The listing builds one solid part. Answer for the finished solid, in the listing's coordinates (mm). A direction names the side the tool comes from. Coordinates: 2 decimals unless noted, no trailing zeros. Loops run counter-clockwise (first coordinate to the right, second up) from the corner with the lowest first, then second, coordinate; pieces in that order, holes last. Notation, with made-up numbers: (33, 72) -> (43, 72) arc R27 ccw to (43, 95) -> close; hole circle Ø2 at (29.25, 46). An arc over 180 degrees is marked (long way). Answer in a Markdown table with one row per item.
```python
from build123d import *

# Parameters (mm, degrees)
F1_DEPTH = 41.95
F3_DEPTH = 39.95
F5_DEPTH = 5


with BuildPart() as f1:
    # F0 (on Front) → F1 (new body)
    with BuildSketch(Plane.XZ):
        Polygon((54.9357536622, -12.7440134094), (54.9357536622, 0.0059865906), (54.9357536622, 12.7559865906), (-52.01294007, 22.7216603247), (-52.0118536268, -22.7213396623), align=None)
    extrude(amount=F1_DEPTH)

    # F2 (on face) → F3 (cut)
    with BuildSketch(Plane.XZ.offset(41.95)):
        Polygon((54.9357536622, 10.7559865906), (-52.0128922544, 20.7216603253), (-52.0119014425, -20.7213396629), (54.9357536622, -10.7440134094), align=None)
    extrude(amount=-F3_DEPTH, mode=Mode.SUBTRACT)

    # F4 (on face) → F5 (cut)
    with BuildSketch(Plane.XZ.offset(2)):
        Polygon((-17.6542899587, 4.4775479473), (-22.824516984, 4.4775479473), (-25.4096304967, 0), (-22.824516984, -4.4775479473), (-17.6542899587, -4.4775479473), (-15.069176446, 0), align=None)
        Polygon((4.0099493481, -2.841678097), (4.4659400954, 2.0518789548), (0.4559907474, 4.8935570518), (-4.0099493481, 2.841678097), (-4.4659400954, -2.0518789548), (-0.4559907474, -4.8935570518), align=None)
        Polygon((24.5754495263, 0.2760817257), (21.8509733677, 4.442849405), (16.8802086264, 4.1667676794), (14.6339200437, -0.2760817257), (17.3583962023, -4.442849405), (22.3291609436, -4.1667676794), align=None)
    extrude(amount=-F5_DEPTH, mode=Mode.SUBTRACT)


solid = f1.part
```
Item 1: A tool of negligible diameter and unlimited length cuts with its end or side. For faces 1 (the face through (1, -41.95, -17)), 2 (the face through (-20, -1, 4.478)), 3 (the face through (0.713, -22.255, -15.803)), from which of +Z, -Z, +X, -X, +Y, -Y can it reach the whole face along a straight path? Write none if from no direction.
Findings below:
| item | result |
|---|---|
| face 1 | +Z, -Z, +X, -X, -Y |
| face 2 | +Y, -Y |
| face 3 | -X, -Y |
Item 2: Determine the mould class of faces 4 (the face through (-4.235, -1.014, 0.429)), 5 (the face through (-1.75, -1.01, 3.88)), 6 (the face through (1, -41.95, 17)), 7 (the face through (0.713, -20.681, -17.803)) for opening direction Z: +Z half, -Z half, draft (parallel to the pull), parting line (faces both ways), or undercut.
Findings below:
| item | result |
|---|---|
| face 4 | undercut |
| face 5 | undercut |
| face 6 | draft |
| face 7 | -Z half |
Item 3: A cutting plane is placed at A-A, the plane y = -18. Determine the outline of the cut face in (x, z), plus the area to 3 significant figures.
Findings below:
| item | result |
|---|---|
| outline | (-52.01, -22.72) -> (54.94, -12.74) -> (54.94, -10.74) -> (-52.01, -20.72) -> close; (-52.01, 20.72) -> (54.94, 10.76) -> (54.94, 12.76) -> (-52.01, 22.72) -> close |
| area | 428 mm2 |
Item 4: Flat-ended cylindrical pins translate along their axes: pin 1 Ø2 at (x, y) = (-20, -1) entering from -Z; pin 2 Ø12 at (x, y) = (21.5, -34) entering from -Z; pin 3 Ø4 at (x, y) = (12.5, -34.5) entering from -Z; pin 4 Ø12 at (y, z) = (-6.5, 9) entering from +X. Find the tip coordinate at first contact, or state that the pin passes through.
Findings below:
| item | result |
|---|---|
| pin 1 | stops at z = -19.83 |
| pin 2 | stops at z = -16.42 |
| pin 3 | stops at z = -16.89 |
| pin 4 | stops at x = 54.94 |
Item 5: A cutting plane is placed at D-D, the plane z = 15.5. Determine the outline of the cut face in (x, y).
Findings below:
| item | result |
|---|---|
| outline | (-52.01, -2) -> (4.02, -2) -> (4.02, -41.95) -> (25.49, -41.95) -> (25.49, 0) -> (-52.01, 0) -> close |
Item 6: A cutting plane is placed at C-C, the plane x = -27.5. Determine the outline of the cut face in (y, z), plus the area to 3 significant figures.
Findings below:
| item | result |
|---|---|
| outline | (-41.95, -20.43) -> (0, -20.43) -> (0, 20.44) -> (-41.95, 20.44) -> (-41.95, 18.44) -> (-2, 18.44) -> (-2, -18.43) -> (-41.95, -18.43) -> close |
| area | 242 mm2 |
Item 7: Find the intervals of material crossed by probe 1 along Z at (x, y) = (37.5, -36); probe 2 along Z at (x, y) = (23.5, -7); probe 3 along Y at (x, z) = (-44, -2), in increasing order.
Findings below:
| item | result |
|---|---|
| probe 1 | z = -14.37 to -12.37, 12.38 to 14.38 |
| probe 2 | z = -15.68 to -13.68, 13.69 to 15.69 |
| probe 3 | y = -2 to 0 |
Item 8: A cutting plane is placed at B-B, the plane x = -2. Determine the outline of the cut face in (y, z), plus the area to 3 significant figures.
Findings below:
| item | result |
|---|---|
| outline | (-41.95, -18.06) -> (0, -18.06) -> (0, -3.8) -> (-2, -3.8) -> (-2, -16.06) -> (-41.95, -16.06) -> close; (-41.95, 16.06) -> (-2, 16.06) -> (-2, 3.77) -> (0, 3.77) -> (0, 18.06) -> (-41.95, 18.06) -> close |
| area | 217 mm2 |
